Input: part model. Units: mm. Frame: model coordinates. A direction names the side the tool comes from. Round coordinates to 2 decimals unless told otherwise and drop trailing zeros. Loops run counter-clockwise (first coordinate to the right, second up) from the corner with the lowest first, then second, coordinate; pieces in that order, holes last. Notation, with made-up numbers: (19.5, 21.25) - (64.5, 21.25) arc R11 cw to (64.5, 26.25) - close; hole circle Ø8 at (71, 85.5). An arc over 180 degrees is marked (long way). One line per question, with ' | ' between items. Start each with the question number.
Item 1: Section D-D, the plane x = 42.5. Return loops of the section in (y, z), plus the area to 3 significant figures.
Item 2: Section C-C, the plane z = 46. Return loops of the section in (x, y).
Item 3: Material intervals for line 1 along Z through (x, y) = (0, 59); line 2 along Y through (x, z) = (38, 22); line 3 along X through (y, z) = (9.5, 19), sorted ascending.
Item 4: First-contact query: pin 1 (2 mm diameter, centred on x = 23.5, z = 29, fed in from +Y); pin 2 (6 mm diameter, centred on y = 46.5, z = 40.5, fed in from -X); pin 3 (1 mm diameter, centred on y = 21, z = -16.5, fed in from -X); pin 4 (12 mm diameter, centred on y = 47, z = 23, fed in from +X). Flat tips, straight axial feed; report the tip coordinate or a pass-through.
Item 5: Set-up query: faces 1 (the face through (-1, 57, -10)), 2 (the face through (-6.86, 9.972, -17.565)), 3 (the face through (5.2, 65, 0.1)). Return all of +Z, -Z, +X, -X, +Y, -Y with unobstructed straight access to the full face (end or side cutting, diameter ignored); none if empty.
Item 6: Section A-A, the plane x = 0. Give the number of separate pieces and of enclosed holes in the cut face, plus the area to 3 significant figures.
Item 7: Section B-B, the plane y = 18. Return loops of the section in (x, z), plus the area to 3 significant figures.
```python
from build123d import *

# Parameters (mm, degrees)
SKETCH1_R           = 52.5
SKETCH1_R_2         = 48.5
BOSS_EXTRUDE1_DEPTH = 65
SKETCH2_R           = 8
SKETCH2_R_2         = 5
BOSS_EXTRUDE2_DEPTH = 65
BOSS_EXTRUDE3_START = -8
BOSS_EXTRUDE3_DEPTH = 4
BOSS_EXTRUDE4_START = -53
BOSS_EXTRUDE4_DEPTH = 4


with BuildPart() as part:
    # Sketch1 → Boss-Extrude1 (new body)
    with BuildSketch(Plane(origin=(0, 0, 0), x_dir=(1, 0, 0), z_dir=(0, 1, 0))):
        Circle(SKETCH1_R)
        Circle(SKETCH1_R_2, mode=Mode.SUBTRACT)
    extrude(amount=BOSS_EXTRUDE1_DEPTH)



with BuildPart() as body_2:
    # Sketch2 → Boss-Extrude2 (new body)
    with BuildSketch(Plane.XZ):
        Circle(SKETCH2_R)
        Circle(SKETCH2_R_2, mode=Mode.SUBTRACT)
    extrude(amount=-BOSS_EXTRUDE2_DEPTH)


with BuildPart() as part_1:
    add(part.part)

    add(body_2.part)  # Boss-Extrude3 merges body 2
    # Sketch2_3 → Boss-Extrude3 (add)
    with BuildSketch(Plane.XZ.offset(BOSS_EXTRUDE3_START)):
        with BuildLine():
            ThreePointArc((0, 8), (4.702282018, 6.472135955), (7.60845213, 2.472135955))
            Line((7.60845213, 2.472135955), (46.12624104, 14.987324227))
            ThreePointArc((46.12624104, 14.987324227), (28.507584736, 39.237324227), (0, 48.5))
            Line((0, 48.5), (0, 8))
        make_face()
        with BuildLine():
            Line((4.498612897, 20.291931451), (7.656121129, 34.53453068))
            ThreePointArc((7.656121129, 34.53453068), (9.081556968, 36.48129187), (11.479516965, 36.748750866))
            ThreePointArc((11.479516965, 36.748750866), (22.629732213, 31.147154283), (31.402773148, 22.273657954))
            ThreePointArc((31.402773148, 22.273657954), (31.889414918, 19.910413097), (30.4784189, 17.953160762))
            Line((30.4784189, 17.953160762), (17.908625798, 10.548986777))
            ThreePointArc((17.908625798, 10.548986777), (15.84479345, 10.183097432), (14.045152036, 11.257606507))
            ThreePointArc((14.045152036, 11.257606507), (10.580134541, 14.562305899), (6.366429359, 16.836525093))
            ThreePointArc((6.366429359, 16.836525093), (4.78839072, 18.216044222), (4.498612897, 20.291931451))
        make_face(mode=Mode.SUBTRACT)
        with BuildLine():
            Line((46.12624104, 14.987324227), (7.60845213, 2.472135955))
            ThreePointArc((7.60845213, 2.472135955), (7.901506725, 1.25147572), (8, 0))
            ThreePointArc((8, 0), (-5.656854249, -5.656854249), (0, 8))
            Line((0, 8), (0, 48.5))
            ThreePointArc((0, 48.5), (-34.294678888, -34.294678888), (48.5, 0))
            ThreePointArc((48.5, 0), (47.902884519, 7.587071554), (46.12624104, 14.987324227))
        make_face()
        with BuildLine():
            Line((8.287843762, -19.060735709), (14.104955724, -32.439177302))
            ThreePointArc((14.104955724, -32.439177302), (14.096031424, -34.851990353), (12.313249487, -36.477854749))
            ThreePointArc((12.313249487, -36.477854749), (0, -38.5), (-12.313249487, -36.477854749))
            ThreePointArc((-12.313249487, -36.477854749), (-14.096031424, -34.851990353), (-14.104955724, -32.439177302))
            Line((-14.104955724, -32.439177302), (-8.287843762, -19.060735709))
            ThreePointArc((-8.287843762, -19.060735709), (-6.83323268, -17.551634794), (-4.745711605, -17.363128214))
            ThreePointArc((-4.745711605, -17.363128214), (0, -18), (4.745711605, -17.363128214))
            ThreePointArc((4.745711605, -17.363128214), (6.83323268, -17.551634794), (8.287843762, -19.060735709))
        make_face(mode=Mode.SUBTRACT)
        with BuildLine():
            Line((-15.566752332, -13.772299075), (-26.492819932, -23.438867123))
            ThreePointArc((-26.492819932, -23.438867123), (-28.790299268, -24.175979847), (-30.887498112, -22.982873197))
            ThreePointArc((-30.887498112, -22.982873197), (-36.615675877, -11.897154283), (-38.497504807, 0.438319126))
            ThreePointArc((-38.497504807, 0.438319126), (-37.502125795, 2.636265233), (-35.21016198, 3.390352984))
            Line((-35.21016198, 3.390352984), (-20.688921471, 1.992116557))
            ThreePointArc((-20.688921471, 1.992116557), (-18.804181667, 1.075037038), (-17.979821767, -0.852061747))
            ThreePointArc((-17.979821767, -0.852061747), (-17.119017293, -5.562305899), (-15.046810695, -9.87894164))
            ThreePointArc((-15.046810695, -9.87894164), (-14.581011618, -11.922543898), (-15.566752332, -13.772299075))
        make_face(mode=Mode.SUBTRACT)
        with BuildLine():
            Line((20.688921471, 1.992116557), (35.21016198, 3.390352984))
            ThreePointArc((35.21016198, 3.390352984), (37.502125795, 2.636265233), (38.497504807, 0.438319126))
            ThreePointArc((38.497504807, 0.438319126), (36.615675877, -11.897154283), (30.887498112, -22.982873197))
            ThreePointArc((30.887498112, -22.982873197), (28.790299268, -24.175979847), (26.492819932, -23.438867123))
            Line((26.492819932, -23.438867123), (15.566752332, -13.772299075))
            ThreePointArc((15.566752332, -13.772299075), (14.581011618, -11.922543898), (15.046810695, -9.87894164))
            ThreePointArc((15.046810695, -9.87894164), (17.119017293, -5.562305899), (17.979821767, -0.852061747))
            ThreePointArc((17.979821767, -0.852061747), (18.804181667, 1.075037038), (20.688921471, 1.992116557))
        make_face(mode=Mode.SUBTRACT)
        with BuildLine():
            Line((-17.908625798, 10.548986777), (-30.4784189, 17.953160762))
            ThreePointArc((-30.4784189, 17.953160762), (-31.889414918, 19.910413097), (-31.402773148, 22.273657954))
            ThreePointArc((-31.402773148, 22.273657954), (-22.629732213, 31.147154283), (-11.479516965, 36.748750866))
            ThreePointArc((-11.479516965, 36.748750866), (-9.081556968, 36.48129187), (-7.656121129, 34.53453068))
            Line((-7.656121129, 34.53453068), (-4.498612897, 20.291931451))
            ThreePointArc((-4.498612897, 20.291931451), (-4.78839072, 18.216044222), (-6.366429359, 16.836525093))
            ThreePointArc((-6.366429359, 16.836525093), (-10.580134541, 14.562305899), (-14.045152036, 11.257606507))
            ThreePointArc((-14.045152036, 11.257606507), (-15.84479345, 10.183097432), (-17.908625798, 10.548986777))
        make_face(mode=Mode.SUBTRACT)
    extrude(amount=-BOSS_EXTRUDE3_DEPTH)

    # Sketch2_4 → Boss-Extrude4 (add)
    with BuildSketch(Plane.XZ.offset(BOSS_EXTRUDE4_START)):
        with BuildLine():
            Line((46.12624104, 14.987324227), (7.60845213, 2.472135955))
            ThreePointArc((7.60845213, 2.472135955), (7.901506725, 1.25147572), (8, 0))
            ThreePointArc((8, 0), (-5.656854249, -5.656854249), (0, 8))
            Line((0, 8), (0, 48.5))
            ThreePointArc((0, 48.5), (-34.294678888, -34.294678888), (48.5, 0))
            ThreePointArc((48.5, 0), (47.902884519, 7.587071554), (46.12624104, 14.987324227))
        make_face()
        with BuildLine():
            Line((8.287843762, -19.060735709), (14.104955724, -32.439177302))
            ThreePointArc((14.104955724, -32.439177302), (14.096031424, -34.851990353), (12.313249487, -36.477854749))
            ThreePointArc((12.313249487, -36.477854749), (0, -38.5), (-12.313249487, -36.477854749))
            ThreePointArc((-12.313249487, -36.477854749), (-14.096031424, -34.851990353), (-14.104955724, -32.439177302))
            Line((-14.104955724, -32.439177302), (-8.287843762, -19.060735709))
            ThreePointArc((-8.287843762, -19.060735709), (-6.83323268, -17.551634794), (-4.745711605, -17.363128214))
            ThreePointArc((-4.745711605, -17.363128214), (0, -18), (4.745711605, -17.363128214))
            ThreePointArc((4.745711605, -17.363128214), (6.83323268, -17.551634794), (8.287843762, -19.060735709))
        make_face(mode=Mode.SUBTRACT)
        with BuildLine():
            Line((-15.566752332, -13.772299075), (-26.492819932, -23.438867123))
            ThreePointArc((-26.492819932, -23.438867123), (-28.790299268, -24.175979847), (-30.887498112, -22.982873197))
            ThreePointArc((-30.887498112, -22.982873197), (-36.615675877, -11.897154283), (-38.497504807, 0.438319126))
            ThreePointArc((-38.497504807, 0.438319126), (-37.502125795, 2.636265233), (-35.21016198, 3.390352984))
            Line((-35.21016198, 3.390352984), (-20.688921471, 1.992116557))
            ThreePointArc((-20.688921471, 1.992116557), (-18.804181667, 1.075037038), (-17.979821767, -0.852061747))
            ThreePointArc((-17.979821767, -0.852061747), (-17.119017293, -5.562305899), (-15.046810695, -9.87894164))
            ThreePointArc((-15.046810695, -9.87894164), (-14.581011618, -11.922543898), (-15.566752332, -13.772299075))
        make_face(mode=Mode.SUBTRACT)
        with BuildLine():
            Line((20.688921471, 1.992116557), (35.21016198, 3.390352984))
            ThreePointArc((35.21016198, 3.390352984), (37.502125795, 2.636265233), (38.497504807, 0.438319126))
            ThreePointArc((38.497504807, 0.438319126), (36.615675877, -11.897154283), (30.887498112, -22.982873197))
            ThreePointArc((30.887498112, -22.982873197), (28.790299268, -24.175979847), (26.492819932, -23.438867123))
            Line((26.492819932, -23.438867123), (15.566752332, -13.772299075))
            ThreePointArc((15.566752332, -13.772299075), (14.581011618, -11.922543898), (15.046810695, -9.87894164))
            ThreePointArc((15.046810695, -9.87894164), (17.119017293, -5.562305899), (17.979821767, -0.852061747))
            ThreePointArc((17.979821767, -0.852061747), (18.804181667, 1.075037038), (20.688921471, 1.992116557))
        make_face(mode=Mode.SUBTRACT)
        with BuildLine():
            Line((-17.908625798, 10.548986777), (-30.4784189, 17.953160762))
            ThreePointArc((-30.4784189, 17.953160762), (-31.889414918, 19.910413097), (-31.402773148, 22.273657954))
            ThreePointArc((-31.402773148, 22.273657954), (-22.629732213, 31.147154283), (-11.479516965, 36.748750866))
            ThreePointArc((-11.479516965, 36.748750866), (-9.081556968, 36.48129187), (-7.656121129, 34.53453068))
            Line((-7.656121129, 34.53453068), (-4.498612897, 20.291931451))
            ThreePointArc((-4.498612897, 20.291931451), (-4.78839072, 18.216044222), (-6.366429359, 16.836525093))
            ThreePointArc((-6.366429359, 16.836525093), (-10.580134541, 14.562305899), (-14.045152036, 11.257606507))
            ThreePointArc((-14.045152036, 11.257606507), (-15.84479345, 10.183097432), (-17.908625798, 10.548986777))
        make_face(mode=Mode.SUBTRACT)
        with BuildLine():
            ThreePointArc((0, 8), (4.702282018, 6.472135955), (7.60845213, 2.472135955))
            Line((7.60845213, 2.472135955), (46.12624104, 14.987324227))
            ThreePointArc((46.12624104, 14.987324227), (28.507584736, 39.237324227), (0, 48.5))
            Line((0, 48.5), (0, 8))
        make_face()
        with BuildLine():
            Line((4.498612897, 20.291931451), (7.656121129, 34.53453068))
            ThreePointArc((7.656121129, 34.53453068), (9.081556968, 36.48129187), (11.479516965, 36.748750866))
            ThreePointArc((11.479516965, 36.748750866), (22.629732213, 31.147154283), (31.402773148, 22.273657954))
            ThreePointArc((31.402773148, 22.273657954), (31.889414918, 19.910413097), (30.4784189, 17.953160762))
            Line((30.4784189, 17.953160762), (17.908625798, 10.548986777))
            ThreePointArc((17.908625798, 10.548986777), (15.84479345, 10.183097432), (14.045152036, 11.257606507))
            ThreePointArc((14.045152036, 11.257606507), (10.580134541, 14.562305899), (6.366429359, 16.836525093))
            ThreePointArc((6.366429359, 16.836525093), (4.78839072, 18.216044222), (4.498612897, 20.291931451))
        make_face(mode=Mode.SUBTRACT)
    extrude(amount=-BOSS_EXTRUDE4_DEPTH)


solid = part_1.part
```
Return value:
1) outline: (0, -30.82) - (65, -30.82) - (65, -23.37) - (57, -23.37) - (57, 23.37) - (65, 23.37) - (65, 30.82) - (0, 30.82) - (0, 23.37) - (8, 23.37) - (8, -23.37) - (0, -23.37) - close; hole (12, -23.37) - (53, -23.37) - (53, 23.37) - (12, 23.37) - close | area: 1,340 mm2
2) outline: (-25.3, 0) - (-15.37, 0) - (-15.37, 8) - (15.37, 8) - (15.37, 0) - (25.3, 0) - (25.3, 65) - (15.37, 65) - (15.37, 57) - (-15.37, 57) - (-15.37, 65) - (-25.3, 65) - close; hole (-15.37, 12) - (15.37, 12) - (15.37, 53) - (-15.37, 53) - close
3) line 1: -52.5 to -48.5, -8 to -5, 5 to 8, 48.5 to 52.5 | line 2: 8 to 12, 53 to 57 | line 3: -48.94 to -31.53, -4.5 to 4.5, 31.53 to 48.94
4) pin 1: through | pin 2: x = -36.74 | pin 3: x = -50 | pin 4: x = 49.67
5) face 1: +Y | face 2: +Y, -Y | face 3: +Z, -Z, +X, -X, +Y
6) separate pieces: 3 | enclosed holes: 1 | area: 1,390 mm2
7) outline: circle Ø105 at (0, 0); circle Ø16 at (0, 0); hole circle Ø97 at (0, 0); hole circle Ø10 at (0, 0) | area: 1,390 mm2
